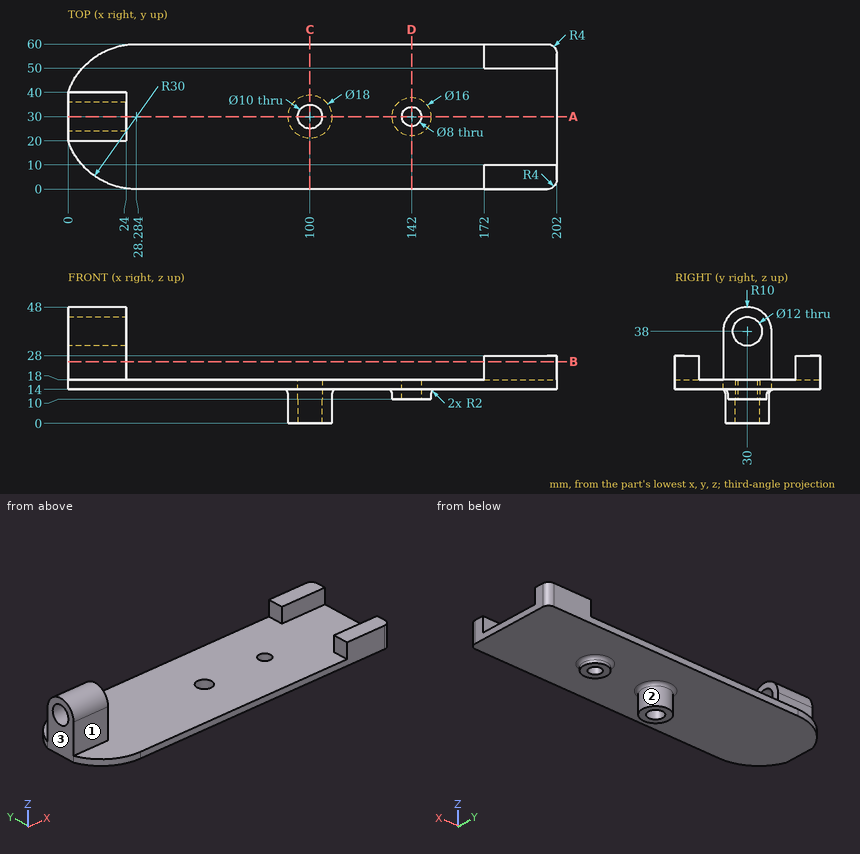
Geometry: see drawing. Coordinates: mm, zero at the bounding-box minimum. A direction names the side the tool comes from. Round coordinates to 2 decimals unless told otherwise and drop trailing zeros. Order: outer loops, then holes, each group sorted by start corner. A loop starts at its lowest first (then second) coordinate and runs counter-clockwise, first axis right, second up. Notation, with made-up numbers: (-28.5, 83) - (18.5, 83) arc R10 cw to (18.5, 98) - close; hole circle Ø7 at (10, 5.5). An arc over 180 degrees is marked (long way). Use a Markdown table: item, result. Add a question column.
1. Set-up query: the marked faces 1, 2 and 3. Return all of +Z, -Z, +X, -X, +Y, -Y with unobstructed straight access to the full face (end or side cutting, diameter ignored); none if empty.
2. Section query A-A (y = 30). Give the number of separate pieces and of enclosed holes in the cut face, then the cut area to 3 significant figures.
3. Section query D-D (x = 142). Return the cut outline in (y, z), then the cut area to 3 significant figures.
4. Section query B-B (z = 25.5). Return the cut outline in (x, y), then the cut area to 3 significant figures.
5. Section query C-C (x = 100). Return the cut outline in (y, z), then the cut area to 3 significant figures.
6. Line query: probe 1 along Y at (x, z) = (100, 6); probe 2 along Y at (x, z) = (100, 14.5); probe 3 along Z at (x, y) = (135, 13). Output: solid intervals per line, ascending.
7. First-contact query: pin 1 (17.5 mm diameter, centred on x = 143.5, y = 32.5, fed in from -Z); pin 2 (6 mm diameter, centred on x = 100, y = 30, fed in from +Z); pin 3 (3 mm diameter, centred on x = 184, y = 56, fed in from +Z); pin 4 (3 mm diameter, centred on x = 56.5, y = 16, fed in from +Z). Flat tips, straight axial feed; report the tip coordinate or a pass-through.
Derived:
| question | item | result |
|---|---|---|
| 1 | face 1 | +Z, +X, -X, -Y |
| 1 | face 2 | -Z |
| 1 | face 3 | +Z, -Z, -X, +Y, -Y |
| 2 | separate pieces | 4 |
| 2 | enclosed holes | 0 |
| 2 | area | 1,320 mm2 |
| 3 | outline | (0, 14) - (20, 14) arc R2 cw to (22, 12) - (22, 10) - (26, 10) - (26, 18) - (0, 18) - close; (34, 10) - (38, 10) - (38, 12) arc R2 cw to (40, 14) - (60, 14) - (60, 18) - (34, 18) - close |
| 3 | area | 242 mm2 |
| 4 | outline | (0, 20) - (24, 20) - (24, 40) - (0, 40) - close; (172, 0) - (198, 0) arc R4 ccw to (202, 4) - (202, 10) - (172, 10) - close; (172, 50) - (202, 50) - (202, 56) arc R4 ccw to (198, 60) - (172, 60) - close |
| 4 | area | 1,070 mm2 |
| 5 | outline | (0, 14) - (19, 14) arc R2 cw to (21, 12) - (21, 0) - (25, 0) - (25, 18) - (0, 18) - close; (35, 0) - (39, 0) - (39, 12) arc R2 cw to (41, 14) - (60, 14) - (60, 18) - (35, 18) - close |
| 5 | area | 314 mm2 |
| 6 | probe 1 | 21 to 25, 35 to 39 |
| 6 | probe 2 | 0 to 25, 35 to 60 |
| 6 | probe 3 | 14 to 18 |
| 7 | pin 1 | z = 10 |
| 7 | pin 2 | through |
| 7 | pin 3 | z = 28 |
| 7 | pin 4 | z = 18 |
